Model file for the job. Use its own axes, mm. A direction names the side the tool comes from. Coordinates: 2 decimals unless noted, no trailing zeros. Loops run counter-clockwise (first coordinate to the right, second up) from the corner with the lowest first, then second, coordinate; pieces in that order, holes last.
from build123d import *

# Parameters (mm, degrees)
SKETCH_1_W      = 60
SKETCH_1_H      = 60
EXTRUDE_1_DEPTH = 30
SKETCH_2_R      = 10
EXTRUDE_2_DEPTH = 15
SKETCH_4_R      = 10
EXTRUDE_3_DEPTH = 15
SKETCH_5_R      = 10
EXTRUDE_4_DEPTH = 15


with BuildPart() as part:
    # 스케치1 → 보스-돌출1 (new body)
    with BuildSketch(Plane(origin=(0, 0, 0), x_dir=(1, 0, 0), z_dir=(0, 1, 0))):
        with Locations((-12.687876758, 2.632618888)):
            Rectangle(SKETCH_1_W, SKETCH_1_H)
    extrude(amount=EXTRUDE_1_DEPTH)

    # 스케치2 → 보스-돌출2 (add)
    with BuildSketch(Plane(origin=(17.312123242, 0, 0), x_dir=(0, 0, -1), z_dir=(1, 0, 0))):
        with Locations((2.632618888, 15)):
            Circle(SKETCH_2_R)
    extrude(amount=EXTRUDE_2_DEPTH)

    # 스케치4 → 보스-돌출3 (add)
    with BuildSketch(Plane.XY.offset(27.367381112)):
        with Locations((-12.687876758, 15)):
            Circle(SKETCH_4_R)
    extrude(amount=EXTRUDE_3_DEPTH)

    # 스케치5 → 보스-돌출4 (add)
    with BuildSketch(Plane(origin=(0, 30, 0), x_dir=(1, 0, 0), z_dir=(0, 1, 0))):
        with Locations(Location((-12.687876758, 2.632618888, 0), (0, 0, 270))):
            Circle(SKETCH_5_R)
    extrude(amount=EXTRUDE_4_DEPTH)


solid = part.part
Q1. Slice it at B-B (z = 2.5). List the corners of the cut face in (x, y), and give its area (3 significant figures).
Answers:
outline: (-42.69, 0) - (17.31, 0) - (17.31, 6.42) - (32.31, 6.42) - (32.31, 23.58) - (17.31, 23.58) - (17.31, 30) - (-4.11, 30) - (-4.11, 45) - (-21.27, 45) - (-21.27, 30) - (-42.69, 30) - close
area: 2,310 mm2
Q2. Flat gauge pins, fed straight in: P1, Ø10, axis at y = 31, z = -24, coming from the +X side; P2, Ø1, axis at x = -2, y = 6.5, coming from the +Z side. Where does each tip first touch, or does it go through?
Answers:
P1: stops at x = 17.31
P2: stops at z = 27.37
Q3. Slice it at A-A (y = 15). List the corners of the cut face in (x, z), and give its area (3 significant figures).
Answers:
outline: (-42.69, -32.63) - (17.31, -32.63) - (17.31, -12.63) - (32.31, -12.63) - (32.31, 7.37) - (17.31, 7.37) - (17.31, 27.37) - (-2.69, 27.37) - (-2.69, 42.37) - (-22.69, 42.37) - (-22.69, 27.37) - (-42.69, 27.37) - close
area: 4,200 mm2
Q4. Which spindle directions (+Z, -Z, +X, -X, +Y, -Y) get a long thin tool onto all of the face, cutting with end or side? Do faces 1 (the flat face through (-13, 15, 42.367)), 2 (the cylindrical face through (-13.99, 24.915, 34.762)), 3 (the flat face through (-42.688, 15, -2)), 4 (the cylindrical face through (-10, 37, 7)), 5 (the cylindrical face through (24.707, 24.915, -1.331)). Say none if no direction does.
Answers:
face 1: +Z, +X, -X, +Y, -Y
face 2: +Z
face 3: +Z, -Z, -X, +Y, -Y
face 4: +Y
face 5: +X
Q5. Slice it at D-D (x = 26). List the corners of the cut face in (y, z).
Answers:
outline: circle Ø20 at (15, -2.63)
Q6. Drill centre lines: line 1 (Z direction, x = -39, y = 29.5); line 2 (X direction, y = 12.5, z = 14.5); line 3 (Y direction, x = -38, z = -28.5). Where is each one in solid material? Low to high.
Answers:
line 1: z = -32.63 to 27.37
line 2: x = -42.69 to 17.31
line 3: y = 0 to 30
Q7. Slice it at C-C (x = 0.5). List the corners of the cut face in (y, z).
Answers:
outline: (0, -32.63) - (30, -32.63) - (30, 27.37) - (0, 27.37) - close
